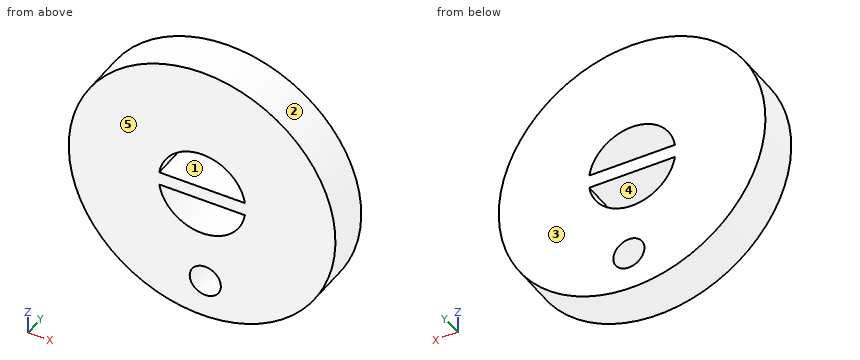
from build123d import *

# Parameters (mm, degrees)
SKETCH1_R           = 6
BOSS_EXTRUDE1_DEPTH = 2
CUT_EXTRUDE1_DEPTH  = 4
SKETCH3_R           = 0.7
CUT_EXTRUDE2_DEPTH  = 4


with BuildPart() as part:
    # Sketch1 → Boss-Extrude1 (new body)
    with BuildSketch(Plane(origin=(0, 0, 0), x_dir=(1, 0, 0), z_dir=(0, 1, 0))):
        with Locations(Location((0, 0, 0), (0, 0, 270))):
            Circle(SKETCH1_R)
    extrude(amount=BOSS_EXTRUDE1_DEPTH)

    # Sketch2 → Cut-Extrude1 (cut)
    with BuildSketch(Plane(origin=(0, 2, 0), x_dir=(1, 0, 0), z_dir=(0, 1, 0))):
        with BuildLine():
            Line((-1.926784887, 0.3), (0, 0.3))
            Line((0, 0.3), (1.926784887, 0.3))
            ThreePointArc((1.926784887, 0.3), (0, 1.95), (-1.926784887, 0.3))
        make_face()
        with BuildLine():
            Line((1.926784887, -0.3), (0, -0.3))
            Line((0, -0.3), (-1.926784887, -0.3))
            ThreePointArc((-1.926784887, -0.3), (0, -1.95), (1.926784887, -0.3))
        make_face()
    extrude(amount=-CUT_EXTRUDE1_DEPTH, mode=Mode.SUBTRACT)

    # Sketch3 → Cut-Extrude2 (cut)
    with BuildSketch(Plane(origin=(0, 2, 0), x_dir=(1, 0, 0), z_dir=(0, 1, 0))):
        with Locations(Location((0.143622542, 4.257382495, 0), (0, 0, 270))):
            Circle(SKETCH3_R)
    extrude(amount=-CUT_EXTRUDE2_DEPTH, mode=Mode.SUBTRACT)


solid = part.part
For this review, take the finished solid that the model builds, in its own axes (mm). Face numbers are marked on the shaded views. A direction names the side the tool comes from. Give positions to 0.01 mm unless a question says otherwise; leave off trailing zeros. Order: outer loops, then holes, each group sorted by start corner. A loop starts at its lowest first (then second) coordinate and runs counter-clockwise, first axis right, second up. Notation, with made-up numbers: M 33,50.5 L 62,50.5 A12 ccw 62,57.5 Z; hole C -3.5,-38.5 d7. An arc over 180 degrees is marked long. Answer in a Markdown table with one row per item. Add a question column.
(1) Consider section B-B on x = 0. State the section outline as (y, z) points, and give its area (3 significant figures).
(2) For the marked faces 4 and 5, list the 3-axis set-ups (+Z, -Z, +X, -X, +Y, -Y) from which the entire face can be reached by the end or side of a thin tool; tool diameter is ignored.
(3) Consider section A-A on x = 1.5. State the section outline as (y, z) points.
(4) Mouldability with a two-part tool opening along Z and no side actions: class the marked faces 1, 2 and 3 as +Z half, -Z half, draft (parallel to the pull), parting line (faces both ways), or undercut.
(5) Consider section D-D on y = 1.3. State the section outline as (x, z) points.
(6) Consider section C-C on z = 1.75. State the section outline as (x, y) points, and give its area (3 significant figures).
(7) For pin 1 (0.8 mm diameter, centred on x = 0.14, z = -4.26, fed in from +Y); pin 2 (0.6 mm diameter, centred on x = -0.5, y = 1, fed in from -Z), all flat-tipped, find the tip position at first contact; note any pin that passes through.
(8) Wall thickness on probe 1 along Z at (x, y) = (0.75, 0.45); probe 2 along Z at (x, y) = (-1.75, 0.45); probe 3 along Z at (x, y) = (0.5, 0.9): over which ranges is each line inside the solid? List them lowest first. Write a range as [from, to].
Evaluation:
| question | item | result |
|---|---|---|
| 1 | outline | M 0,-6 L 2,-6 L 2,-4.94 L 0,-4.94 Z; M 0,-3.57 L 2,-3.57 L 2,-1.95 L 0,-1.95 Z; M 0,-0.3 L 2,-0.3 L 2,0.3 L 0,0.3 Z; M 0,1.95 L 2,1.95 L 2,6 L 0,6 Z |
| 1 | area | 14.7 mm^2 |
| 2 | face 4 | +Y, -Y |
| 2 | face 5 | +Z, -Z, +X, -X, -Y |
| 3 | outline | M 0,-5.81 L 2,-5.81 L 2,-1.25 L 0,-1.25 Z; M 0,-0.3 L 2,-0.3 L 2,0.3 L 0,0.3 Z; M 0,1.25 L 2,1.25 L 2,5.81 L 0,5.81 Z |
| 4 | face 1 | undercut |
| 4 | face 2 | parting line |
| 4 | face 3 | draft |
| 5 | outline | C 0,0 d12; hole M -1.93,-0.3 A1.95 ccw 1.93,-0.3 Z; hole M -1.93,0.3 L 1.93,0.3 A1.95 ccw Z; hole C 0.14,-4.26 d1.4 |
| 6 | outline | M -5.74,0 L -0.86,0 L -0.86,2 L -5.74,2 Z; M 0.86,0 L 5.74,0 L 5.74,2 L 0.86,2 Z |
| 6 | area | 19.5 mm^2 |
| 7 | pin 1 | passes through |
| 7 | pin 2 | stops at z = -6 |
| 8 | probe 1 | z = [-5.95, -4.61], [-3.91, -1.8], [-0.3, 0.3], [1.8, 5.95] |
| 8 | probe 2 | z = [-5.74, -0.86], [-0.3, 0.3], [0.86, 5.74] |
| 8 | probe 3 | z = [-5.98, -4.86], [-3.65, -1.88], [-0.3, 0.3], [1.88, 5.98] |
